Job drawing, mm, ordinate dimensions from the low corner. One solid piece. Coordinates: 2 decimals unless noted, no trailing zeros. Write each loop counter-clockwise with the first axis right and the second up, starting at its lowest first coordinate (ties: lowest second). Pieces come first, ordered by that corner, then holes.
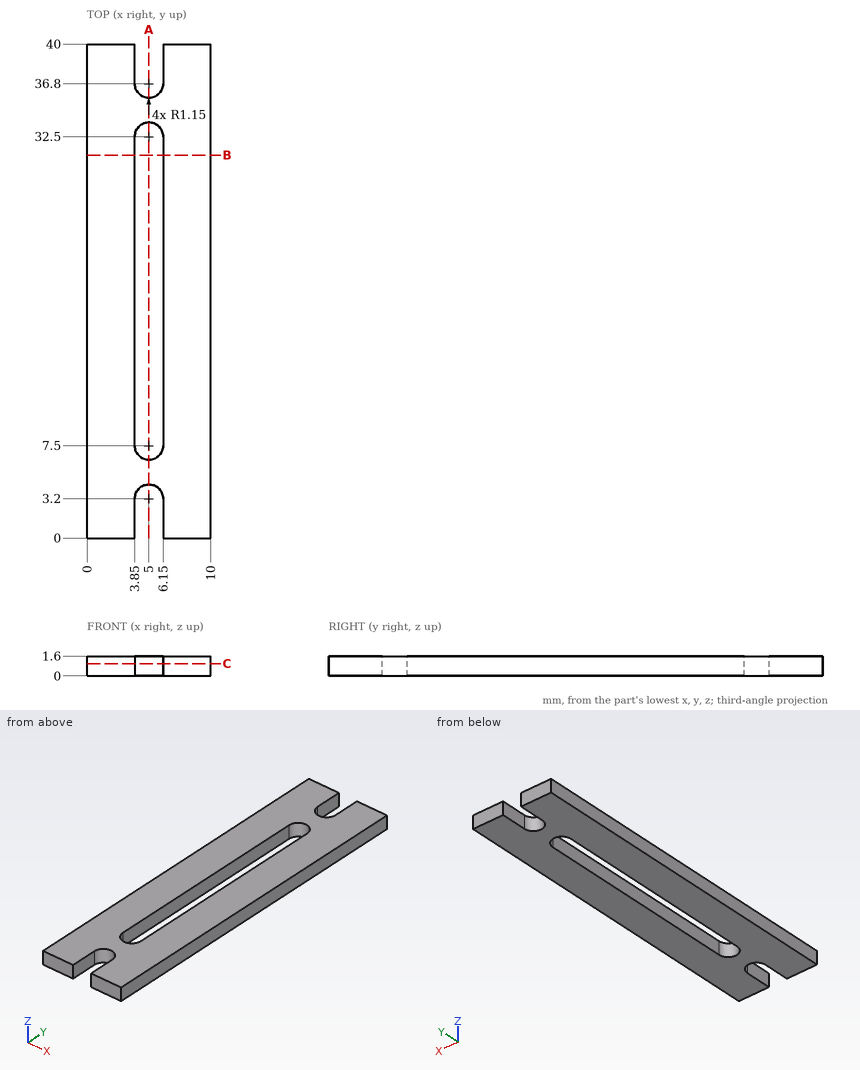
1. Saw through at B-B on y = 31. List the corners of the cut face in (x, z).
Computed values:
outline: (0, 0) - (3.85, 0) - (3.85, 1.6) - (0, 1.6) - close; (6.15, 0) - (10, 0) - (10, 1.6) - (6.15, 1.6) - close
2. Saw through at A-A on x = 5. List the corners of the cut face in (y, z), plus the area to 3 significant figures.
Computed values:
outline: (4.35, 0) - (6.35, 0) - (6.35, 1.6) - (4.35, 1.6) - close; (33.65, 0) - (35.65, 0) - (35.65, 1.6) - (33.65, 1.6) - close
area: 6.40 mm2
3. Saw through at C-C on z = 1. List the corners of the cut face in (x, y), plus the area to 3 significant figures.
Computed values:
outline: (0, 0) - (3.85, 0) - (3.85, 3.2) arc R1.15 cw to (6.15, 3.2) - (6.15, 0) - (10, 0) - (10, 40) - (6.15, 40) - (6.15, 36.8) arc R1.15 cw to (3.85, 36.8) - (3.85, 40) - (0, 40) - close; hole (3.85, 7.5) arc R1.15 ccw to (6.15, 7.5) - (6.15, 32.5) arc R1.15 ccw to (3.85, 32.5) - close
area: 319 mm2
4. Probe line 1 along X through (y, z) = (15, 1.2); line 2 along Y through (x, z) = (5, 0.2); line 3 along Y through (x, z) = (4, 0.65). List the from-to ranges inside material, lowest first.
Computed values:
line 1: x = 0 to 3.85, 6.15 to 10
line 2: y = 4.35 to 6.35, 33.65 to 35.65
line 3: y = 3.77 to 6.93, 33.07 to 36.23
